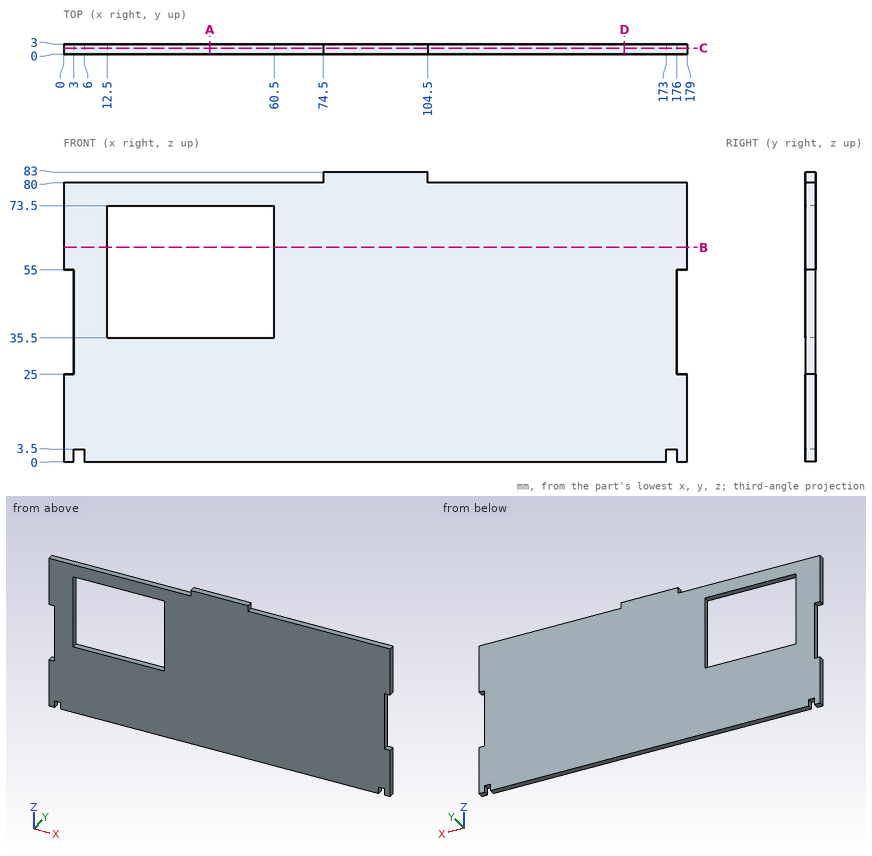
Can you work these out from the drawing? Everything is in mm from the part's minimum corner. Give positions to 0.01 mm unless a question says otherwise; leave off trailing zeros. Order: outer loops, then holes, each group sorted by start corner. A loop starts at its lowest first (then second) coordinate and runs counter-clockwise, first axis right, second up.
Item 1: If we section it at B-B, the plane z = 61.5: Write out the boundary of the cut face in (x, y).
Item 2: If we section it at D-D, the plane x = 161: Write out the boundary of the cut face in (y, z).
Item 3: I need wall thicknesses on line 1 (X direction, y = 1.8, z = 43); line 2 (Z direction, x = 53.5, y = 0.8); line 3 (X direction, y = 2.8, z = 68.5). Which ranges of each line are inside material? Lowest first, please.
Item 4: I'm going to push flat-ended pins straight in: pin 1 (1.5 mm diameter, centred on x = 2, y = 2, fed in from +Z); pin 2 (0.9 mm diameter, centred on y = 1, z = 35, fed in from +X); pin 3 (1.5 mm diameter, centred on x = 4, y = 2, fed in from -Z). Where does each tip first touch, or does it pass through?
Item 5: If we section it at C-C, the plane y = 1.85: Write out the boundary of the cut face in (x, z), plus the area to 3 significant figures.
Item 6: If we section it at A-A, the plane x = 42: Write out the boundary of the cut face in (y, z), plus the area to 3 significant figures.
Values:
1. outline: (0, 0) - (12.5, 0) - (12.5, 3) - (0, 3) - close; (60.5, 0) - (179, 0) - (179, 3) - (60.5, 3) - close
2. outline: (0, 0) - (3, 0) - (3, 80) - (0, 80) - close
3. line 1: x = 3 to 12.5, 60.5 to 176
3. line 2: z = 0 to 35.5, 73.5 to 80
3. line 3: x = 0 to 12.5, 60.5 to 179
4. pin 1: stops at z = 80
4. pin 2: stops at x = 176
4. pin 3: stops at z = 3.5
5. outline: (0, 0) - (3, 0) - (3, 3.5) - (6, 3.5) - (6, 0) - (173, 0) - (173, 3.5) - (176, 3.5) - (176, 0) - (179, 0) - (179, 25) - (176, 25) - (176, 55) - (179, 55) - (179, 80) - (104.5, 80) - (104.5, 83) - (74.5, 83) - (74.5, 80) - (0, 80) - (0, 55) - (3, 55) - (3, 25) - (0, 25) - close; hole (12.5, 35.5) - (60.5, 35.5) - (60.5, 73.5) - (12.5, 73.5) - close
5. area: 12,400 mm2
6. outline: (0, 0) - (3, 0) - (3, 35.5) - (0, 35.5) - close; (0, 73.5) - (3, 73.5) - (3, 80) - (0, 80) - close
6. area: 126 mm2
